Input: part model. Units: mm. Frame: model coordinates. Face numbers are marked on the shaded views. Coordinates: 2 decimals unless noted, no trailing zeros. Order: outer loops, then holes, each group sorted by start corner. A loop starts at its lowest first (then second) coordinate and runs counter-clockwise, first axis right, second up. Notation, with made-up numbers: (-10.5, 8) -> (46.5, 8) arc R37 ccw to (46.5, 45) -> close; hole circle Ø6 at (20, 67.5). An arc over 180 degrees is marked (long way). Answer as CSV lines item,"result".
from build123d import *

# Parameters (mm, degrees)
SKETCH1_W           = 150
SKETCH1_H           = 90
BOSS_EXTRUDE1_DEPTH = 10
SKETCH2_W           = 49.6
SKETCH2_H           = 9.9
BOSS_EXTRUDE2_DEPTH = 9
SKETCH4_W           = 138
SKETCH4_H           = 58
CUT_EXTRUDE1_DEPTH  = 7
FILLET1_R           = 5


with BuildPart() as part:
    # Sketch1 → Boss-Extrude1 (new body)
    with BuildSketch(Plane(origin=(0, 0, 0), x_dir=(1, 0, 0), z_dir=(0, 1, 0))):
        with Locations((75, 45)):
            Rectangle(SKETCH1_W, SKETCH1_H)
    extrude(amount=BOSS_EXTRUDE1_DEPTH)

    # Sketch2 → Boss-Extrude2 (add)
    with BuildSketch(Plane.XZ):
        with Locations((75, -4.95)):
            Rectangle(SKETCH2_W, SKETCH2_H)
        with Locations((75, -85.05)):
            Rectangle(SKETCH2_W, SKETCH2_H)
    extrude(amount=BOSS_EXTRUDE2_DEPTH)

    # Sketch4 → Cut-Extrude1 (cut)
    with BuildSketch(Plane.XZ):
        with Locations((75, -45)):
            Rectangle(SKETCH4_W, SKETCH4_H)
    extrude(amount=-CUT_EXTRUDE1_DEPTH, mode=Mode.SUBTRACT)

    # Fillet1
    # the kernel refuses this fillet: 5 mm, written as the material it takes off along each edge
    with BuildSketch(Plane(origin=(112.3, -9, -80.1), x_dir=(0, 1, 0), z_dir=(-1, 0, 0)), Plane(origin=(37.7, -9, -90), x_dir=(0, 1, 0), z_dir=(1, 0, 0)), Plane(origin=(112.3, -9, -9.9), x_dir=(0, 0, 1), z_dir=(-1, 0, 0))) as fillet1_piece_1:
        with BuildLine():
            CenterArc((FILLET1_R, FILLET1_R), FILLET1_R, 180, 90)
            Line((0, FILLET1_R), (0, 0))
            Line((0, 0), (FILLET1_R, 0))
        make_face()
    extrude(amount=74.6, mode=Mode.SUBTRACT)
    with BuildSketch(Plane(origin=(37.7, -9, 0), x_dir=(0, 1, 0), z_dir=(1, 0, 0))) as fillet1_piece_2:
        with BuildLine():
            CenterArc((FILLET1_R, -FILLET1_R), FILLET1_R, 90, 90)
            Line((0, -FILLET1_R), (0, 0))
            Line((0, 0), (FILLET1_R, 0))
        make_face()
    extrude(amount=74.6, mode=Mode.SUBTRACT)
    with BuildSketch(Plane(origin=(150, 10, 12.5), x_dir=(-1, 0, 0), z_dir=(0, 0, -1))) as fillet1_piece_3:
        with BuildLine():
            CenterArc((FILLET1_R, -FILLET1_R), FILLET1_R, 90, 90)
            Line((0, -FILLET1_R), (0, 0))
            Line((0, 0), (FILLET1_R, 0))
        make_face()
    extrude(amount=115, mode=Mode.SUBTRACT)
    with BuildSketch(Plane(origin=(162.5, 10, -90), x_dir=(0, 0, 1), z_dir=(-1, 0, 0))) as fillet1_piece_4:
        with BuildLine():
            CenterArc((FILLET1_R, -FILLET1_R), FILLET1_R, 90, 90)
            Line((0, -FILLET1_R), (0, 0))
            Line((0, 0), (FILLET1_R, 0))
        make_face()
    extrude(amount=175, mode=Mode.SUBTRACT)
    with BuildSketch(Plane(origin=(-12.5, 10, 0), x_dir=(0, -1, 0), z_dir=(1, 0, 0))) as fillet1_piece_5:
        with BuildLine():
            CenterArc((FILLET1_R, FILLET1_R), FILLET1_R, 180, 90)
            Line((0, FILLET1_R), (0, 0))
            Line((0, 0), (FILLET1_R, 0))
        make_face()
    extrude(amount=175, mode=Mode.SUBTRACT)
    with BuildSketch(Plane(origin=(0, 10, -102.5), x_dir=(0, -1, 0), z_dir=(0, 0, 1))) as fillet1_piece_6:
        with BuildLine():
            CenterArc((FILLET1_R, FILLET1_R), FILLET1_R, 180, 90)
            Line((0, FILLET1_R), (0, 0))
            Line((0, 0), (FILLET1_R, 0))
        make_face()
    extrude(amount=115, mode=Mode.SUBTRACT)


solid = part.part
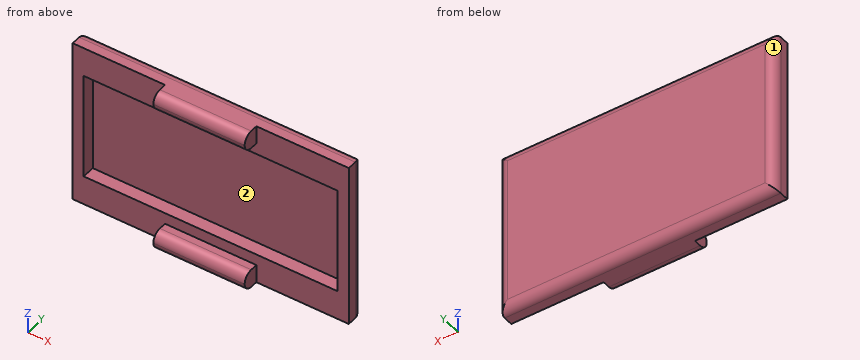
1. Mould query, pull axis Z, two halves, no side actions, for the marked faces 1 and 2. Classes: released by +Z, released by -Z, zero draft, split by the parting line, or undercut.
Findings:
face 1,"zero draft"
face 2,"undercut"
2. Cut plane A-A (y = -5.5). Return the cut outline in (x, z).
Findings:
outline,"(50.2, -89.77) -> (99.8, -89.77) -> (99.8, -80.33) -> (50.2, -80.33) -> close; (50.2, -9.67) -> (99.8, -9.67) -> (99.8, -0.23) -> (50.2, -0.23) -> close"
3. Contact query for flat-ended pins moving along their axis: pin 1 (4.5 mm diameter, centred on y = -3.5, z = -3.5, fed in from -X); pin 2 (2.5 mm diameter, centred on y = -2.5, z = -82.5, fed in from +X). Output: stop coordinate, or through.
Findings:
pin 1,"stops at x = 50.2"
pin 2,"stops at x = 99.8"
4. Cut plane C-C (z = -34). Return the cut outline in (x, y).
Findings:
outline,"(0, 0) -> (6, 0) -> (6, 7) -> (144, 7) -> (144, 0) -> (150, 0) -> (150, 5) arc R5 ccw to (145, 10) -> (5, 10) arc R5 ccw to (0, 5) -> close"
5. Cut plane D-D (x = 62.5). Return the cut outline in (y, z), plus the area to 3 significant figures.
Findings:
outline,"(-9, -85.05) arc R5 ccw to (-4, -90) -> (5, -90) arc R5 ccw to (10, -85) -> (10, -5) arc R5 ccw to (5, 0) -> (-4, 0) arc R5 ccw to (-9, -4.95) arc R5 ccw to (-4, -9.9) -> (0, -9.9) -> (0, -16) -> (7, -16) -> (7, -74) -> (0, -74) -> (0, -80.1) -> (-4, -80.1) arc R5 ccw to start"
area,"640 mm2"
6. Cut plane B-B (x = 116.5). Return the cut outline in (y, z), plus the area to 3 significant figures.
Findings:
outline,"(0, -90) -> (5, -90) arc R5 ccw to (10, -85) -> (10, -5) arc R5 ccw to (5, 0) -> (0, 0) -> (0, -16) -> (7, -16) -> (7, -74) -> (0, -74) -> close"
area,"483 mm2"
7. Ray query, line 1 along X through (y, z) = (0.75, -29); line 2 along Z through (x, y) = (95.5, -1.75); line 3 along Z through (x, y) = (118, 2.75). Return the intervals inside material, ascending.
Findings:
line 1,"x = 0 to 6, 144 to 150"
line 2,"z = -90 to -80.1, -9.9 to 0"
line 3,"z = -90 to -74, -16 to 0"
